```python
from build123d import *

# Parameters (mm, degrees)
IZIM1_W                     = 110
IZIM1_H                     = 87
Y_KSEKLIK_EKSTR_ZYON1_DEPTH = 3
RADYUS1_R                   = 2
IZIM2_R                     = 1.5
IZIM2_R_2                   = 1.25
KES_EKSTR_ZYON1_DEPTH       = 10


with BuildPart() as part:
    # Çizim1 → Yükseklik-Ekstrüzyon1 (new body)
    with BuildSketch(Plane(origin=(0, 0, 0), x_dir=(1, 0, 0), z_dir=(0, 1, 0))):
        Rectangle(IZIM1_W, IZIM1_H)
    extrude(amount=Y_KSEKLIK_EKSTR_ZYON1_DEPTH)

    # Radyus1
    radyus1_edges = [part.edges().sort_by_distance(p)[0] for p in [
        (55, 1.5, 43.5),
        (-55, 1.5, 43.5),
        (-55, 1.5, -43.5),
        (55, 1.5, -43.5),
    ]]
    fillet(radyus1_edges, radius=RADYUS1_R)

    # Çizim2 → Kes-Ekstrüzyon1 (cut)
    with BuildSketch(Plane(origin=(0, 3, 0), x_dir=(1, 0, 0), z_dir=(0, 1, 0))):
        with Locations(Location((-18.5, 40.5, 0), (0, 0, 270))):
            Circle(IZIM2_R)
        with Locations(Location((18.5, 40.5, 0), (0, 0, 270))):
            Circle(IZIM2_R)
        with Locations(Location((18.5, 3.5, 0), (0, 0, 270))):
            Circle(IZIM2_R)
        with Locations(Location((-18.5, 3.5, 0), (0, 0, 270))):
            Circle(IZIM2_R)
        with Locations(Location((-42, 27.54, 0), (0, 0, 270))):
            Circle(IZIM2_R_2)
        with Locations(Location((-42, 9.54, 0), (0, 0, 270))):
            Circle(IZIM2_R_2)
        with Locations(Location((42, 27.54, 0), (0, 0, 270))):
            Circle(IZIM2_R_2)
        with Locations(Location((42, 9.54, 0), (0, 0, 270))):
            Circle(IZIM2_R_2)
        with Locations(Location((-16, -36.58, 0), (0, 0, 270))):
            Circle(IZIM2_R)
        with Locations(Location((-16, -16.5, 0), (0, 0, 270))):
            Circle(IZIM2_R)
        with Locations(Location((16, -16.5, 0), (0, 0, 270))):
            Circle(IZIM2_R)
        with Locations(Location((16, -36.58, 0), (0, 0, 270))):
            Circle(IZIM2_R)
    extrude(amount=-KES_EKSTR_ZYON1_DEPTH, mode=Mode.SUBTRACT)


solid = part.part
```
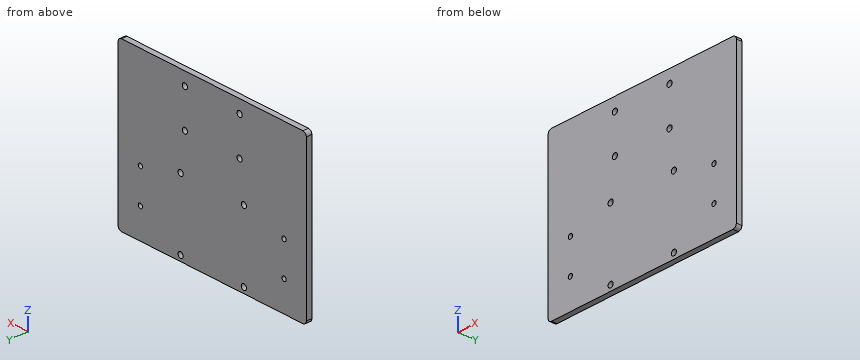
Can you work these out from the model? Positions are in its coordinate system, mm. Round coordinates to 2 decimals unless told otherwise and drop trailing zeros. Loops run counter-clockwise (first coordinate to the right, second up) from the corner with the lowest first, then second, coordinate; pieces in that order, holes last. Notation, with made-up numbers: M 63.25,-5.75 L 104.25,-5.75 A18 ccw 104.25,6.25 Z; hole C 88.5,63.25 d5. An arc over 180 degrees is marked long. Write item = value, one per line. Start each with the question number.
(1) I'm going to push a flat-ended pin straight in: P1, Ø2, axis at x = 42, z = -9.54, coming from the +Y side. Where does the tip first touch, or does it pass through?
(2) I need wall thicknesses on line 1 along X through (y, z) = (2.05, 36.58); line 2 along X through (y, z) = (2, -3.5); line 3 along Z through (x, y) = (-42.5, 2.2). Which ranges of each line are inside material? Lowest first, please.
(3) Suppose I cut it at A-A on z = -9.54. Write out the boundary of the cut face in (x, y).
(4) Suppose I cut it at B-B on x = 42. Write out the boundary of the cut face in (y, z), plus the area to 3 significant figures.
Answer block:
q1.P1 = through
q2.line_1 = -55 to -17.5, -14.5 to 14.5, 17.5 to 55
q2.line_2 = -55 to -20, -17 to 17, 20 to 55
q2.line_3 = -43.5 to -28.69, -26.39 to -10.69, -8.39 to 43.5
q3.outline = M -55,0 L -43.25,0 L -43.25,3 L -55,3 Z; M -40.75,0 L 40.75,0 L 40.75,3 L -40.75,3 Z; M 43.25,0 L 55,0 L 55,3 L 43.25,3 Z
q4.outline = M 0,-43.5 L 3,-43.5 L 3,-28.79 L 0,-28.79 Z; M 0,-26.29 L 3,-26.29 L 3,-10.79 L 0,-10.79 Z; M 0,-8.29 L 3,-8.29 L 3,43.5 L 0,43.5 Z
q4.area = 246 mm²
